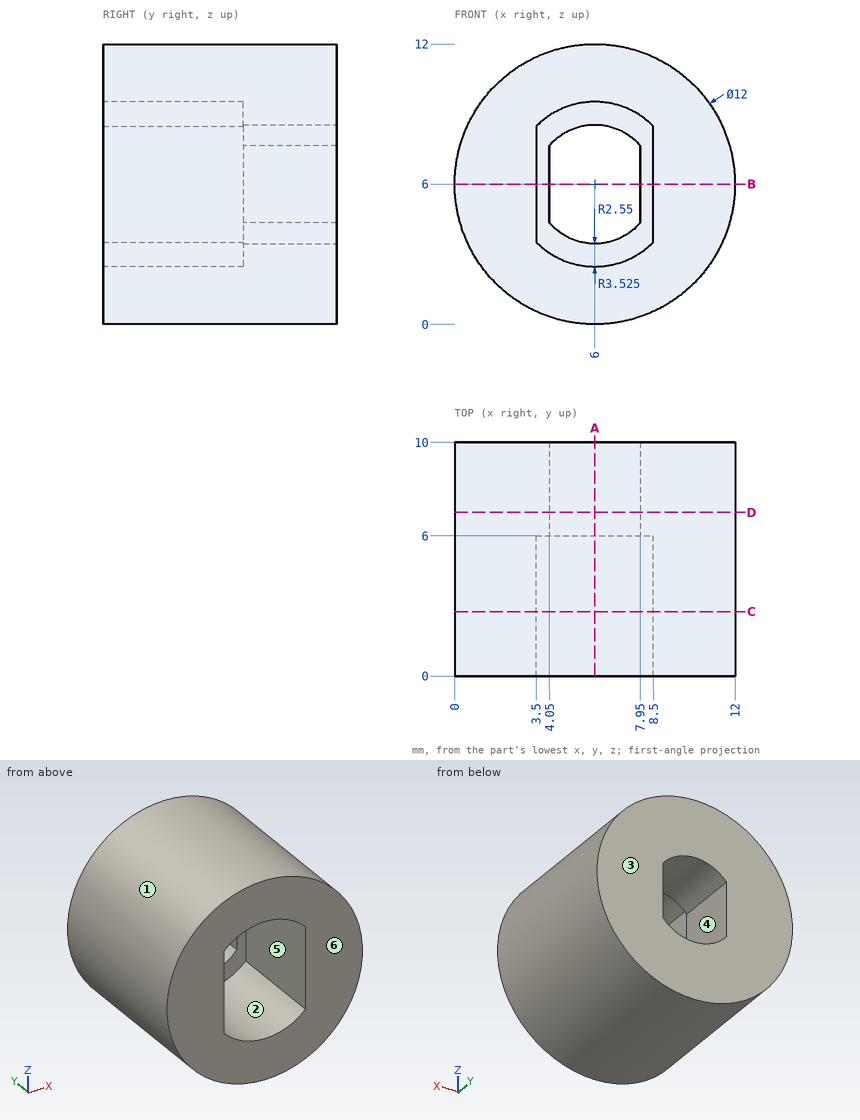
Geometry: see drawing. Coordinates: mm, zero at the bounding-box minimum. A direction names the side the tool comes from. Round coordinates to 2 decimals unless told otherwise and drop trailing zeros. Loops run counter-clockwise (first coordinate to the right, second up) from the corner with the lowest first, then second, coordinate; pieces in that order, holes last. Notation, with made-up numbers: (50, 66) -> (83, 66) arc R11 ccw to (83, 74) -> close; hole circle Ø5 at (-1.75, 5). An arc over 180 degrees is marked (long way). Use one line per item in the form item = value. Start each with the question number.
Item 1: Section query D-D on y = 7. Return the cut outline in (x, z).
Item 2: Section query C-C on y = 2.75. Return the cut outline in (x, z) (3 decimals), then the cut area to 3 significant figures.
Item 3: Section query A-A on x = 6. Return the cut outline in (y, z) (3 decimals), then the cut area to 3 significant figures.
Item 4: Section query B-B on z = 6. Return the cut outline in (x, y), then the cut area to 3 significant figures.
Item 5: Mould query, pull axis X, two halves, no side actions, for the marked faces 1, 2 and 3. Classes: pulls with the +X half, pulls with the -X half, needs draft (parallel to the pull), parting line crosses it, or undercut.
Item 6: Material intervals for L1, parallel to X at y = 4.5, z = 6; L2, parallel to Z at x = 4.5, y = 8.5; L3, parallel to X at y = 3, z = 8.5, sorted ascending. Write a range as from..to.
Item 7: Contact query for flat-ended pins moving along their axis: pin 1 Ø1 at (y, z) = (8.5, 3.5) entering from -X; pin 2 Ø3 at (x, y) = (2.5, 8) entering from +Z; pin 3 Ø2.5 at (x, z) = (5, 4.5) entering from -Y. Output: stop coordinate, or through.
Item 8: Set-up query: the marked faces 4, 5 and 6. Return all of +Z, -Z, +X, -X, +Y, -Y with unobstructed straight access to the full face (end or side cutting, diameter ignored); none if empty.
Ans:
q1.outline = circle Ø12 at (6, 6); hole (4.05, 4.36) arc R2.55 ccw to (7.95, 4.36) -> (7.95, 7.64) arc R2.55 ccw to (4.05, 7.64) -> close
q2.outline = circle Ø12 at (6, 6); hole (3.5, 3.515) arc R3.525 ccw to (8.5, 3.515) -> (8.5, 8.485) arc R3.525 ccw to (3.5, 8.485) -> close
q2.area = 81.1 mm^2
q3.outline = (0, 0) -> (10, 0) -> (10, 3.45) -> (6, 3.45) -> (6, 2.475) -> (0, 2.475) -> close; (0, 9.525) -> (6, 9.525) -> (6, 8.55) -> (10, 8.55) -> (10, 12) -> (0, 12) -> close
q3.area = 57.3 mm^2
q4.outline = (0, 0) -> (3.5, 0) -> (3.5, 6) -> (4.05, 6) -> (4.05, 10) -> (0, 10) -> close; (7.95, 6) -> (8.5, 6) -> (8.5, 0) -> (12, 0) -> (12, 10) -> (7.95, 10) -> close
q4.area = 74.4 mm^2
q5.face_1 = parting line crosses it
q5.face_2 = undercut
q5.face_3 = needs draft
q6.L1 = 0..3.5, 8.5..12
q6.L2 = 0.19..3.94, 8.06..11.81
q6.L3 = 0.55..3.51, 8.49..11.45
q7.pin_1 = 0.34
q7.pin_2 = 11.66
q7.pin_3 = 6
q8.face_4 = +Y, -Y
q8.face_5 = -Y
q8.face_6 = +Z, -Z, +X, -X, -Y
